Input: part model. Units: mm. Frame: model coordinates. A direction names the side the tool comes from. Coordinates: 2 decimals unless noted, no trailing zeros. Loops run counter-clockwise (first coordinate to the right, second up) from the corner with the lowest first, then second, coordinate; pieces in that order, holes last.
(1) Line query: L1, parallel to X at y = -28, z = 1.3; L2, parallel to Y at x = 47, z = 1.65; L3, parallel to X at y = -6, z = 2.75. Output: solid intervals per line, ascending.
(2) Section C-C, the plane x = 47. Return loops of the section in (y, z).
(3) Mould query, pull axis Y, two halves, no side actions, for faces 1 (the face through (-1, 35, 1)), 2 (the face through (-1, -35, 1)), 3 (the face through (-77, 5, 2)), 4 (the face through (-1, 24, 3)). Classes: released by +Y, released by -Y, zero draft, split by the parting line, or undercut.
(4) Set-up query: faces 5 (the face through (-78, 0, 2)), 6 (the face through (81.5, 0, 1)). Return all of +Z, -Z, +X, -X, +Y, -Y with unobstructed straight access to the full face (end or side cutting, diameter ignored); none if empty.
(5) Section D-D, the plane y = 8. Return loops of the section in (x, z), then the cut area to 3 significant figures.
(6) Contact query for a flat-ended pin moving along its axis: P1, Ø1.8, axis at x = -47, y = 28, coming from the -Z side. Output: stop coordinate, or through.
(7) Section B-B, the plane y = 28. Return loops of the section in (x, z), then the cut area to 3 significant figures.
(8) Section A-A, the plane z = 0.95. Return loops of the section in (x, y), then the cut area to 3 significant figures.
```python
from build123d import *

# Parameters (mm, degrees)
SKETCH1_W               = 163
SKETCH1_H               = 70
BOSS_EXTRUDE1_DEPTH     = 3
SKETCH2_W               = 2.7
SKETCH2_H               = 10
CUT_EXTRUDE1_DEPTH      = 3
CUT_EXTRUDE2_REACH      = 5
SKETCH3_W               = 100
SKETCH3_H               = 40
SKETCH4_R               = 1.5
CUT_EXTRUDE3_DEPTH      = 3
MIRROR3_COPY_1_SKETCH_R = 1.5
MIRROR3_COPY_1_DEPTH    = 3


with BuildPart() as part:
    # Sketch1 → Boss-Extrude1 (new body)
    with BuildSketch(Plane.XY):
        Rectangle(SKETCH1_W, SKETCH1_H)
    extrude(amount=BOSS_EXTRUDE1_DEPTH)

    # Sketch2 → Cut-Extrude1 (cut)
    with BuildSketch(Plane.XY.offset(3)):
        with Locations((-76.65, 0)):
            Rectangle(SKETCH2_W, SKETCH2_H)
    cut_extrude1 = extrude(amount=-CUT_EXTRUDE1_DEPTH, mode=Mode.SUBTRACT)

    # Mirror1: Cut-Extrude1 across plane
    add(cut_extrude1.mirror(Plane(origin=(0, 0, 0), x_dir=(0, 0, 1), z_dir=(1, 0, 0))), mode=Mode.SUBTRACT)

    # Sketch3 → Cut-Extrude2 (cut, up to next)
    with BuildSketch(Plane.XY.offset(3), mode=Mode.PRIVATE) as cut_extrude2_sk1:
        Rectangle(SKETCH3_W, SKETCH3_H)
    cut_extrude2_tool1 = extrude(cut_extrude2_sk1.sketch, amount=-CUT_EXTRUDE2_REACH, mode=Mode.PRIVATE) & part.part
    add(cut_extrude2_tool1.solids().sort_by_distance((0, 0, 3))[0], mode=Mode.SUBTRACT)

    # Sketch4 → Cut-Extrude3 (cut)
    with BuildSketch(Plane.XY.offset(3)):
        with Locations((47, 28)):
            Circle(SKETCH4_R)
    cut_extrude3 = extrude(amount=-CUT_EXTRUDE3_DEPTH, mode=Mode.SUBTRACT)

    # Mirror2: Cut-Extrude3 across plane
    add(cut_extrude3.mirror(Plane(origin=(0, 0, 0), x_dir=(0, 0, 1), z_dir=(1, 0, 0))), mode=Mode.SUBTRACT)

    # Mirror3: Cut-Extrude3 across plane
    add(cut_extrude3.mirror(Plane.ZX), mode=Mode.SUBTRACT)

    # Mirror3 copy 1 sketch → Mirror3 copy 1 (cut)
    with BuildSketch(Plane(origin=(0, 0, 3), x_dir=(-1, 0, 0), z_dir=(0, 0, 1))):
        with Locations((47, 28)):
            Circle(MIRROR3_COPY_1_SKETCH_R)
    extrude(amount=-MIRROR3_COPY_1_DEPTH, mode=Mode.SUBTRACT)


solid = part.part
```
Report:
1. L1: x = -81.5 to -48.5, -45.5 to 45.5, 48.5 to 81.5
1. L2: y = -35 to -29.5, -26.5 to -20, 20 to 26.5, 29.5 to 35
1. L3: x = -81.5 to -50, 50 to 81.5
2. outline: (-35, 0) - (-29.5, 0) - (-29.5, 3) - (-35, 3) - close; (-26.5, 0) - (-20, 0) - (-20, 3) - (-26.5, 3) - close; (20, 0) - (26.5, 0) - (26.5, 3) - (20, 3) - close; (29.5, 0) - (35, 0) - (35, 3) - (29.5, 3) - close
3. face 1: released by +Y
3. face 2: released by -Y
3. face 3: undercut
3. face 4: zero draft
4. face 5: +Z, -Z
4. face 6: +Z, -Z, +X, +Y, -Y
5. outline: (-81.5, 0) - (-50, 0) - (-50, 3) - (-81.5, 3) - close; (50, 0) - (81.5, 0) - (81.5, 3) - (50, 3) - close
5. area: 189 mm2
6. P1: passes through
7. outline: (-81.5, 0) - (-48.5, 0) - (-48.5, 3) - (-81.5, 3) - close; (-45.5, 0) - (45.5, 0) - (45.5, 3) - (-45.5, 3) - close; (48.5, 0) - (81.5, 0) - (81.5, 3) - (48.5, 3) - close
7. area: 471 mm2
8. outline: (-81.5, -35) - (81.5, -35) - (81.5, 35) - (-81.5, 35) - close; hole (-78, -5) - (-75.3, -5) - (-75.3, 5) - (-78, 5) - close; hole (-50, -20) - (50, -20) - (50, 20) - (-50, 20) - close; hole circle Ø3 at (-47, -28); hole circle Ø3 at (-47, 28); hole circle Ø3 at (47, -28); hole circle Ø3 at (47, 28); hole (75.3, -5) - (78, -5) - (78, 5) - (75.3, 5) - close
8. area: 7,330 mm2
